```python
from build123d import *

# Parameters (mm, degrees)
CHANFREIN1_SIZE = 1.5


with BuildPart() as part:
    # Esquisse1 → Révolution1 (revolve)
    with BuildSketch(Plane.XY, mode=Mode.PRIVATE) as r_volution1_sk:
        Polygon((0, 10), (0, 18.425), (27.5, 18.425), (27.5, 23), (34.5, 23), (34.5, 10), align=None)
    revolve(r_volution1_sk.sketch.rotate(Axis((-4.444335788, 0, 0), (1, 0, 0)), 90), axis=Axis((-4.444335788, 0, 0), (1, 0, 0)))  # turned: the seam where the file's is

    # Chanfrein1
    chanfrein1_edges = [part.edges().sort_by_distance(p)[0] for p in [
        (0, 0, -18.425),
        (0, 0, -10),
        (34.5, 0, -10),
        (34.5, 0, -23),
    ]]
    chamfer(chanfrein1_edges, length=CHANFREIN1_SIZE)


solid = part.part
```
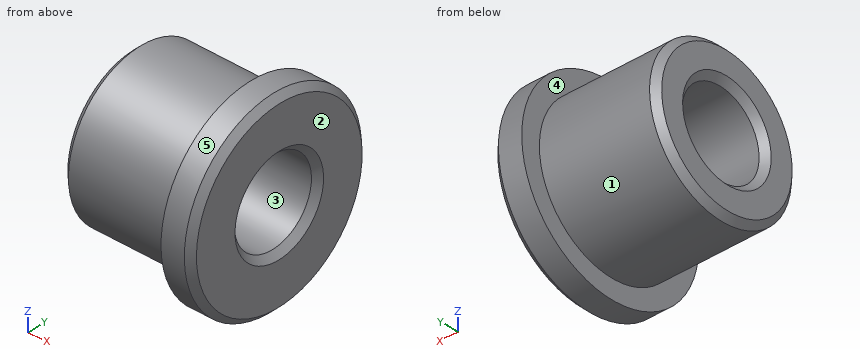
The model under review builds one solid part; all positions refer to its coordinate system, in mm. Face numbers are marked on the shaded views. A direction names the side the tool comes from. Coordinates: 2 decimals unless noted, no trailing zeros. Write each loop counter-clockwise with the first axis right and the second up, starting at its lowest first coordinate (ties: lowest second). Pieces come first, ordered by that corner, then holes. Notation, with made-up numbers: (37.5, 14) -> (43.5, 14) arc R24 ccw to (43.5, 29) -> close; hole circle Ø9 at (0, 15.25). An arc over 180 degrees is marked (long way). One line per item, written item: value. Start each with the question number.
Q1. Add section C-C, the plane x = 31. Give the boundary of the cut face in (y, z), then the cut area to 3 significant figures.
Q2. For the marked faces 4 and 5, list the 3-axis set-ups (+Z, -Z, +X, -X, +Y, -Y) from which the entire face can be reached by the end or side of a thin tool; tool diameter is ignored.
Q3. To check wall thickness, follow probe 1 along Y at (x, z) = (24.5, 0.5); probe 2 along Y at (x, z) = (2, -4); probe 3 along X at (y, z) = (17, 8). State the ranges of each line that lie inside material, in increasing order.
Q4. Add section D-D, the plane x = 19. Give the boundary of the cut face in (y, z) (3 decimals), then the cut area to 3 significant figures.
Q5. Clearance check with flat-ended pins moving along their axes: P1, Ø8, axis at x = 7.5, z = 12, coming from the -Y side; P2, Ø12, axis at x = 20, z = 3, coming from the +Y side (3 decimals); P3, Ø3, axis at x = 16.5, y = 6, coming from the +Z side. State where each tip first meets the part, or that it passes through.
Q6. Add section A-A, the plane z = 0. Give the boundary of the cut face in (x, y) (3 decimals).
Q7. The part is to be moulded in two halves that separate along Y. For the marked faces 1, 2 and 3, say which applies: +Y half, -Y half, draft (parallel to the pull), parting line (faces both ways), or undercut.
Response:
1. outline: circle Ø46 at (0, 0); hole circle Ø20 at (0, 0)
1. area: 1,350 mm²
2. face 4: -X
2. face 5: +X, -X
3. probe 1: -18.42 to -9.99, 9.99 to 18.42
3. probe 2: -17.99 to -9.17, 9.17 to 17.99
3. probe 3: 27.5 to 34.5
4. outline: circle Ø36.85 at (0, 0); hole circle Ø20 at (0, 0)
4. area: 752 mm²
5. P1: y = -16.6
5. P2: y = 18.425
5. P3: z = 17.87
6. outline: (0, -16.925) -> (1.5, -18.425) -> (27.5, -18.425) -> (27.5, -23) -> (33, -23) -> (34.5, -21.5) -> (34.5, -11.5) -> (33, -10) -> (1.5, -10) -> (0, -11.5) -> close; (0, 11.5) -> (1.5, 10) -> (33, 10) -> (34.5, 11.5) -> (34.5, 21.5) -> (33, 23) -> (27.5, 23) -> (27.5, 18.425) -> (1.5, 18.425) -> (0, 16.925) -> close
7. face 1: parting line
7. face 2: draft
7. face 3: undercut
